```python
from build123d import *

# Parameters (mm, degrees)
ESQUISSE1_R        = 17
BOSS_EXTRU_1_DEPTH = 3.4
ESQUISSE2_R        = 19.8
ESQUISSE2_R_2      = 17
BOSS_EXTRU_2_DEPTH = 0.8


with BuildPart() as part:
    # Esquisse1 → Boss.-Extru.1 (new body)
    with BuildSketch(Plane.XY):
        with BuildLine():
            Line((10.604819554, 19.085304433), (10.844597942, 19.490397698))
            ThreePointArc((10.844597942, 19.490397698), (11.465620902, 19.951920532), (12.230041829, 19.832197983))
            ThreePointArc((12.230041829, 19.832197983), (0, -23.3), (-12.230041829, 19.832197983))
            ThreePointArc((-12.230041829, 19.832197983), (-11.465620902, 19.951920532), (-10.844597942, 19.490397698))
            Line((-10.844597942, 19.490397698), (-10.604819554, 19.085304433))
            ThreePointArc((-10.604819554, 19.085304433), (-8.050510374, 18.285863427), (-6.988397979, 20.74259267))
            Line((-6.988397979, 20.74259267), (-10.6, 31.462358462))
            ThreePointArc((-10.6, 31.462358462), (-7.615939872, 32.314663233), (-4.565333975, 32.884612294))
            Line((-4.565333975, 32.884612294), (-3.426014723, 24.718632018))
            ThreePointArc((-3.426014723, 24.718632018), (-3.621264858, 23.974046302), (-4.287669622, 23.58877342))
            ThreePointArc((-4.287669622, 23.58877342), (-5.278203354, 20.042601197), (-2.038983016, 21.793014323))
            Line((-2.038983016, 21.793014323), (-3.1, 33.054954243))
            ThreePointArc((-3.1, 33.054954243), (0, 33.2), (3.1, 33.054954243))
            Line((3.1, 33.054954243), (2.038983016, 21.793014323))
            ThreePointArc((2.038983016, 21.793014323), (5.278203354, 20.042601197), (4.287669622, 23.58877342))
            ThreePointArc((4.287669622, 23.58877342), (3.621264858, 23.974046302), (3.426014723, 24.718632018))
            Line((3.426014723, 24.718632018), (4.565333975, 32.884612294))
            ThreePointArc((4.565333975, 32.884612294), (7.615939872, 32.314663233), (10.6, 31.462358462))
            Line((10.6, 31.462358462), (6.988397979, 20.74259267))
            ThreePointArc((6.988397979, 20.74259267), (8.050510374, 18.285863427), (10.604819554, 19.085304433))
        make_face()
        Circle(ESQUISSE1_R, mode=Mode.SUBTRACT)
    extrude(amount=BOSS_EXTRU_1_DEPTH)

    # Esquisse2 → Boss.-Extru.2 (add)
    with BuildSketch(Plane.XY.offset(3.4)):
        Circle(ESQUISSE2_R)
        Circle(ESQUISSE2_R_2, mode=Mode.SUBTRACT)
    extrude(amount=BOSS_EXTRU_2_DEPTH)


solid = part.part
```
Build history of the part. All positions in model axes, mm. A direction names the side the tool comes from. Round coordinates to 2 decimals unless told otherwise and drop trailing zeros. Write each loop counter-clockwise with the first axis right and the second up, starting at its lowest first coordinate (ties: lowest second). Pieces come first, ordered by that corner, then holes.
1) Band-saw the part on D-D, the plane y = -19. List the corners of the cut face in (x, z), and give its area (3 significant figures).
2) Band-saw the part on C-C, the plane z = 2. List the corners of the cut face in (x, y), and give its area (3 significant figures).
3) Band-saw the part on A-A, the plane y = 0. List the corners of the cut face in (x, z), and give its area (3 significant figures).
4) Pin check, flat tips, straight feed: pin 1 (10 mm diameter, centred on x = 8, y = -9, fed in from -Z); pin 2 (2.5 mm diameter, centred on x = 4.03, y = 21.61, fed in from +Z); pin 3 (1 mm diameter, centred on x = 9, z = 2.5, fed in from -Y). Stop position of each tip, or through.
5) Drill centre lines: probe 1 along Y at (x, z) = (5, 2.55); probe 2 along X at (y, z) = (20.5, 3.15); probe 3 along X at (y, z) = (26, 1.8). Where is each one in solid material? Low to high.
6) Mould opens along Y. For faces 1 (the cylindrical face through (-11.476, 19.955, 1.676)), 2 (the cylindrical face through (-8.09, 18.27, 1.68)), 3 (the flat face through (2, 20, 3.4)), 4 (the cylindrical face through (5.226, 20.003, 1.676)) say: +Y half, -Y half, draft (parallel to the pull), parting line (faces both ways), or undercut.
7) 3-axis set-ups, long thin cutter, end or side, ignore diameter. For faces 5 (the flat face through (8.82, 26.18, 1.68)), 6 (the flat face through (-4.004, 28.859, 1.676)), 7 (the cylindrical face through (3.6, 24, 1.7)): which of +Z, -Z, +X, -X, +Y, -Y reach the whole face in a straight line?
8) Band-saw the part on B-B, the plane x = 0. List the corners of the cut face in (y, z).
Ans:
1. outline: (-13.49, 0) - (13.49, 0) - (13.49, 3.4) - (5.57, 3.4) - (5.57, 4.2) - (-5.57, 4.2) - (-5.57, 3.4) - (-13.49, 3.4) - close
1. area: 101 mm2
2. outline: (-12.23, 19.83) arc R23.3 ccw (long way) to (12.23, 19.83) arc R1 ccw to (10.84, 19.49) - (10.6, 19.09) arc R2 cw to (6.99, 20.74) - (10.6, 31.46) arc R33.2 ccw to (4.57, 32.88) - (3.43, 24.72) arc R1 ccw to (4.29, 23.59) arc R2 cw (long way) to (2.04, 21.79) - (3.1, 33.05) arc R33.2 ccw to (-3.1, 33.05) - (-2.04, 21.79) arc R2 cw (long way) to (-4.29, 23.59) arc R1 ccw to (-3.43, 24.72) - (-4.57, 32.88) arc R33.2 ccw to (-10.6, 31.46) - (-6.99, 20.74) arc R2 cw to (-10.6, 19.09) - (-10.84, 19.49) arc R1 ccw to start; hole circle Ø34 at (0, 0)
2. area: 905 mm2
3. outline: (-23.3, 0) - (-17, 0) - (-17, 4.2) - (-19.8, 4.2) - (-19.8, 3.4) - (-23.3, 3.4) - close; (17, 0) - (23.3, 0) - (23.3, 3.4) - (19.8, 3.4) - (19.8, 4.2) - (17, 4.2) - close
3. area: 47.3 mm2
4. pin 1: stops at z = 0
4. pin 2: passes through
4. pin 3: stops at y = -21.69
5. probe 1: y = -22.76 to -16.25, 16.25 to 19.86, 23.35 to 32.82
5. probe 2: x = -6.92 to -5.7, -2.36 to 2.36, 5.7 to 6.92
5. probe 3: x = -8.76 to -3.6, -2.44 to 2.44, 3.6 to 8.76
6. face 1: +Y half
6. face 2: undercut
6. face 3: draft
6. face 4: undercut
7. face 5: +Z, -Z, +X
7. face 6: +Z, -Z, +Y
7. face 7: +Z, -Z
8. outline: (-23.3, 0) - (-17, 0) - (-17, 4.2) - (-19.8, 4.2) - (-19.8, 3.4) - (-23.3, 3.4) - close; (17, 0) - (33.2, 0) - (33.2, 3.4) - (19.8, 3.4) - (19.8, 4.2) - (17, 4.2) - close
